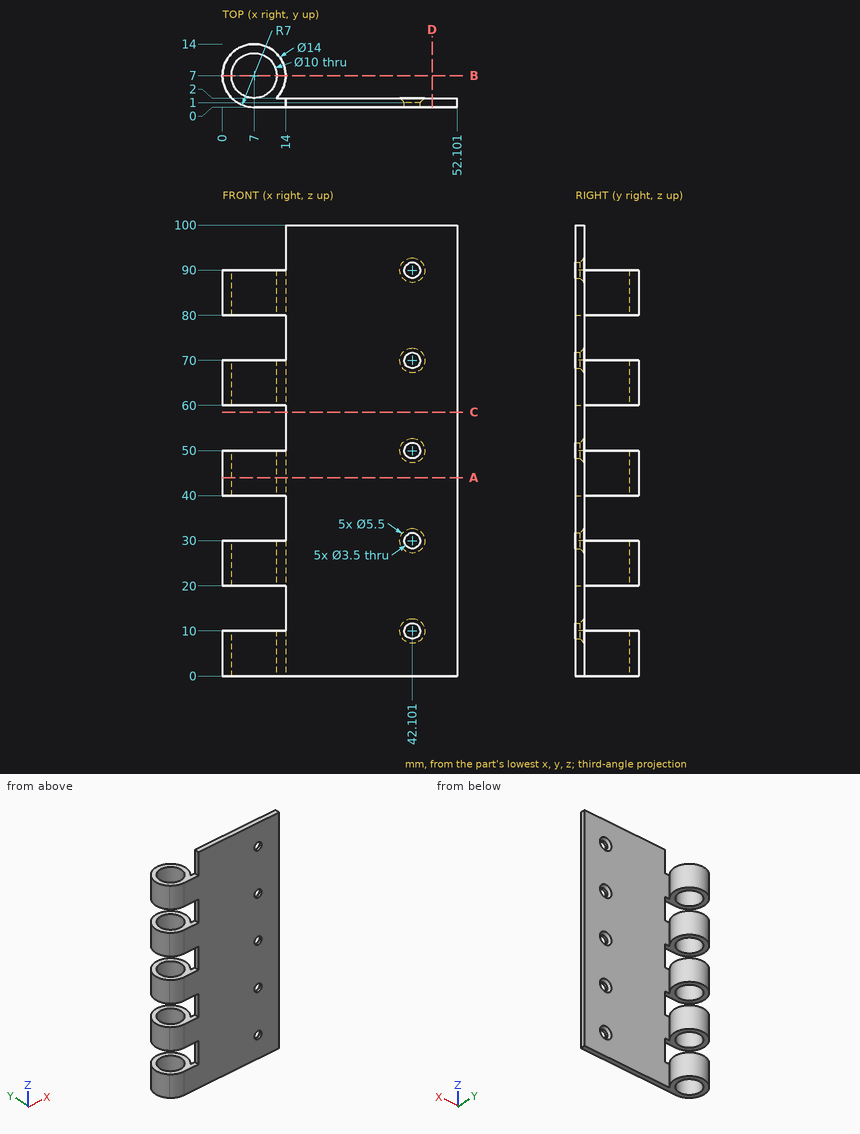
Geometry: see drawing. Coordinates: mm, zero at the bounding-box minimum. Coordinates: 2 decimals unless noted, no trailing zeros. Loops run counter-clockwise (first coordinate to the right, second up) from the corner with the lowest first, then second, coordinate; pieces in that order, holes last.
Q1. Cut plane D-D (x = 46.5). Output: boundary loops of the cut face in (y, z), then the cut area to 3 significant figures.
Q2. Cut plane B-B (y = 7). Give the number of separate pieces and of enclosed holes in the cut face, then the cut area to 3 significant figures.
Q3. Cut plane C-C (z = 58.5). Output: boundary loops of the cut face in (x, y), then the cut area to 3 significant figures.
Q4. Material intervals for line 1 (Z direction, x = 12, y = 5.5); line 2 (Y direction, x = 40, z = 73.5); line 3 (X direction, y = 1, z = 77), sorted ascending.
Q5. Contact query for flat-ended pins moving along their axis: pin 1 (3 mm diameter, centred on x = 42.1, z = 70, fed in from -Y); pin 2 (1.6 mm diameter, centred on y = 1, z = 34, fed in from -X); pin 3 (7 mm diameter, centred on x = 8.5, y = 6.5, fed in from +Z); pin 4 (2 mm diameter, centred on y = 9, z = 88.5, fed in from +X). Output: stop coordinate, or through.
Q6. Cut plane A-A (z = 44). Output: boundary loops of the cut face in (x, y), then the cut area to 3 significant figures.
Working result:
1. outline: (0, 0) - (2, 0) - (2, 100) - (0, 100) - close
1. area: 200 mm2
2. separate pieces: 10
2. enclosed holes: 0
2. area: 200 mm2
3. outline: (14, 0) - (52.1, 0) - (52.1, 2) - (14, 2) - close
3. area: 76.2 mm2
4. line 1: z = 0 to 10, 20 to 30, 40 to 50, 60 to 70, 80 to 90
4. line 2: y = 0 to 2
4. line 3: x = 14 to 52.1
5. pin 1: passes through
5. pin 2: stops at x = 14
5. pin 3: stops at z = 90
5. pin 4: stops at x = 13.93
6. outline: (7, 0) - (52.1, 0) - (52.1, 2) - (11.9, 2) arc R7 ccw (long way) to start; hole circle Ø10 at (7, 7)
6. area: 159 mm2
